Here's how the part is built. I have some questions about the finished solid (model axes, mm). Face numbers are marked on the shaded views. A direction names the side the tool comes from. Coordinates: 2 decimals unless noted, no trailing zeros. Order: outer loops, then holes, each group sorted by start corner. A loop starts at its lowest first (then second) coordinate and runs counter-clockwise, first axis right, second up. Notation, with made-up numbers: (-21, -27) - (11, -27) arc R29 cw to (11, 1) - close; hole circle Ø5 at (55.5, -13). An arc over 180 degrees is marked (long way). Use CSV: the item, a comma, the result in double quotes. Start each with the question number.
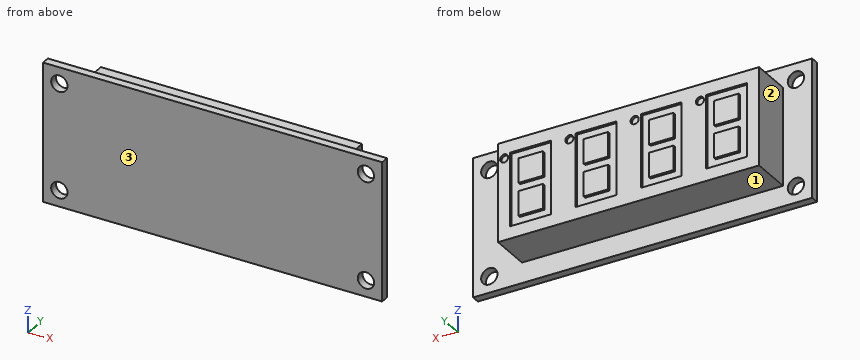
from build123d import *

# Parameters (mm, degrees)
SKETCH1_W           = 66
SKETCH1_H           = 27
SKETCH1_R           = 1.5875
BOSS_EXTRUDE1_DEPTH = 1.5875
SKETCH2_W           = 50.8
SKETCH2_H           = 19.05
BOSS_EXTRUDE2_DEPTH = 7.9375
SKETCH3_R           = 0.79375
SKETCH3_W           = 7.9375
SKETCH3_H           = 14.2875
SKETCH3_W_2         = 4.7625
SKETCH3_H_2         = 4.7625
CUT_EXTRUDE1_DEPTH  = 0.5
LPATTERN1_COUNT     = 4
LPATTERN1_PITCH     = 12.7


with BuildPart() as part:
    # Sketch1 → Boss-Extrude1 (new body)
    with BuildSketch(Plane(origin=(0, 0, 0), x_dir=(1, 0, 0), z_dir=(0, 1, 0))):
        with Locations((33, 13.5)):
            Rectangle(SKETCH1_W, SKETCH1_H)
        with Locations((62.825, 23.825)):
            Circle(SKETCH1_R, mode=Mode.SUBTRACT)
        with Locations((3.175, 23.825)):
            Circle(SKETCH1_R, mode=Mode.SUBTRACT)
        with Locations((3.175, 3.175)):
            Circle(SKETCH1_R, mode=Mode.SUBTRACT)
        with Locations((62.825, 3.175)):
            Circle(SKETCH1_R, mode=Mode.SUBTRACT)
    extrude(amount=BOSS_EXTRUDE1_DEPTH)

    # Sketch2 → Boss-Extrude2 (add)
    with BuildSketch(Plane(origin=(0, 1.5875, 0), x_dir=(1, 0, 0), z_dir=(0, 1, 0))):
        with Locations((31.075, 13.5)):
            Rectangle(SKETCH2_W, SKETCH2_H)
    extrude(amount=BOSS_EXTRUDE2_DEPTH)

    # Sketch3 → Cut-Extrude1 (cut)
    with BuildSketch(Plane(origin=(0, 9.525, 0), x_dir=(1, 0, 0), z_dir=(0, 1, 0))):
        with Locations((17.184375, 7.15)):
            Circle(SKETCH3_R)
        with Locations((12.025, 13.5)):
            Rectangle(SKETCH3_W, SKETCH3_H)
        with Locations((12.025, 16.675)):
            Rectangle(SKETCH3_W_2, SKETCH3_H_2, mode=Mode.SUBTRACT)
        with Locations((12.025, 10.325)):
            Rectangle(SKETCH3_W_2, SKETCH3_H_2, mode=Mode.SUBTRACT)
    cut_extrude1 = extrude(amount=-CUT_EXTRUDE1_DEPTH, mode=Mode.SUBTRACT)

    # LPattern1: Cut-Extrude1 ×4
    with Locations(*[(i * LPATTERN1_PITCH, 0, 0) for i in range(1, LPATTERN1_COUNT)]):
        add(cut_extrude1, mode=Mode.SUBTRACT)


solid = part.part
Item 1: Suppose I cut it at D-D on y = 1. Write out the boundary of the cut face in (x, z) (1 decimal), then the cut area to 3 significant figures.
Item 2: For pin 1 Ø1 at (x, y) = (22, 2) entering from +Z; pin 2 Ø4 at (x, z) = (62.825, -23.825) entering from +Y; pin 3 Ø2.5 at (x, y) = (27, 5) entering from -Z (3 decimals); pin 4 Ø5 at (x, y) = (56, 4.5) entering from +Z (3 decimals), each with a flat end and sliding along its axis, tell me the tip position at first contact or that it passes through.
Item 3: Suppose I cut it at B-B on x = 9. Write out the boundary of the cut face in (y, z) (1 decimal).
Item 4: Please list where these lines run through material, in increasing order: line 1 along X through (y, z) = (1, -24.75); line 2 along Z through (x, y) = (62, 1.5); line 3 along Y through (x, z) = (15, -17.25) (3 decimals). Write a range as from..to.
Item 5: Suppose I cut it at A-A on z = -21.25. Write out the boundary of the cut face in (x, y) (1 decimal).
Item 6: For the marked faces 1, 2 and 3, which set-ups out of +Z, -Z, +X, -X, +Y, -Y let a thin tool reach every point of the face, with its end or its side?
Item 7: Suppose I cut it at C-C on z = -24.5. Write out the boundary of the cut face in (x, y).
Here are the results:
1,outline,"(0, -27) - (66, -27) - (66, 0) - (0, 0) - close; hole circle Ø3.2 at (3.2, -23.8); hole circle Ø3.2 at (3.2, -3.2); hole circle Ø3.2 at (62.8, -23.8); hole circle Ø3.2 at (62.8, -3.2)"
1,area,"1,750 mm^2"
2,pin 1,"z = 0"
2,pin 2,"y = 1.59"
2,pin 3,"z = -23.025"
2,pin 4,"z = -3.975"
3,outline,"(0, -27) - (1.6, -27) - (1.6, -23) - (9.5, -23) - (9.5, -20.6) - (9, -20.6) - (9, -6.4) - (9.5, -6.4) - (9.5, -4) - (1.6, -4) - (1.6, 0) - (0, 0) - close"
4,line 1,"0..1.88, 4.47..61.53, 64.12..66"
4,line 2,"-27..-25.18, -22.47..-4.53, -1.82..0"
4,line 3,"0..9.025"
5,outline,"(0, 0) - (66, 0) - (66, 1.6) - (56.5, 1.6) - (56.5, 9.5) - (5.7, 9.5) - (5.7, 1.6) - (0, 1.6) - close"
6,face 1,"-Z, +X, -X, +Y"
6,face 2,"+Z, -Z, -X, +Y"
6,face 3,"+Z, -Z, +X, -X, -Y"
7,outline,"(0, 0) - (1.74, 0) - (1.74, 1.59) - (0, 1.59) - close; (4.61, 0) - (61.39, 0) - (61.39, 1.59) - (4.61, 1.59) - close; (64.26, 0) - (66, 0) - (66, 1.59) - (64.26, 1.59) - close"
